The listing builds one solid part. Answer for the finished solid, in the listing's coordinates (mm). Face numbers are marked on the shaded views. A direction names the side the tool comes from. Round coordinates to 2 decimals unless told otherwise and drop trailing zeros. Loops run counter-clockwise (first coordinate to the right, second up) from the corner with the lowest first, then second, coordinate; pieces in that order, holes last. Notation, with made-up numbers: (38, 62.25) -> (45, 62.25) arc R31 ccw to (45, 99.25) -> close; hole circle Ø9 at (52.5, 72). An arc over 180 degrees is marked (long way). Use a Markdown table: item, result. Add a question column.
Q1. Section A-A on y = 25 is taken. Give the vertices of the cut face in (x, z).
Q2. For a pull along Y with two mould halves and no side action, classify the marked faces 1, 2 and 3 as released by +Y, released by -Y, zero draft, split by the parting line, or undercut.
Q3. Which of the six approach directions +Z, -Z, +X, -X, +Y, -Y give full straight-line access (tool end or side, diameter ignored) to the marked faces 4 and 5?
Q4. Consider line 1 (Y direction, x = 25, z = 22); line 2 (X direction, y = 27.5, z = 4); line 3 (X direction, y = 20, z = 5.5). Determine where each line is inside the solid, lowest interval first.
Q5. Given pin 1 Ø13.5 at (x, y) = (138.5, 74) entering from -Z; pin 2 Ø2 at (x, y) = (180, 52.5) entering from -Z; pin 3 Ø4 at (x, z) = (122.5, 8) entering from +Y; pin 4 Ø13 at (x, y) = (25, 25) entering from -Z, each flat-ended and moving along its own axis, determine where each tip first touches the part or whether it passes through.
Q6. Section C-C on x = 105 is taken. Give the vertices of the cut face in (y, z), then the cut area to 3 significant figures.
Q7. Section D-D on x = 25 is taken. Give the vertices of the cut face in (y, z).
Q8. Section B-B on z = 24.5 is taken. Give the vertices of the cut face in (x, y), then the cut area to 3 significant figures.
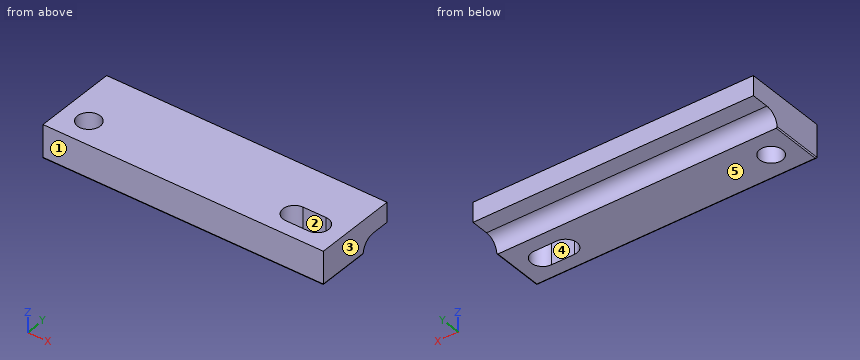
from build123d import *

# Parameters (mm, degrees)
SKETCH_1_W          = 270
SKETCH_1_H          = 80
EXTRUDE_1_DEPTH     = 32
SKETCH_2_R          = 11
CUT_EXTRUDE_1_DEPTH = 284.414890223
CUT_EXTRUDE_2_DEPTH = 284.414890223
FILLET_1_R          = 1
FILLET_2_R          = 1
FILLET_4_R          = 1


with BuildPart() as part:
    # 草图1 → 拉伸1 (new body)
    with BuildSketch(Plane.XY):
        with Locations((135, 40)):
            Rectangle(SKETCH_1_W, SKETCH_1_H)
    extrude(amount=EXTRUDE_1_DEPTH)

    # 草图2 → 切除-拉伸1 (cut, through all)
    with BuildSketch(Plane.XY.offset(32)):
        with Locations((25, 25)):
            Circle(SKETCH_2_R)
        with BuildLine():
            Line((223, 36), (245, 36))
            ThreePointArc((245, 36), (256, 25), (245, 14))
            Line((245, 14), (223, 14))
            ThreePointArc((223, 14), (212, 25), (223, 36))
        make_face()
    extrude(amount=-CUT_EXTRUDE_1_DEPTH, mode=Mode.SUBTRACT)

    # 草图3 → 切除-拉伸2 (cut, through all)
    with BuildSketch(Plane.ZY):
        with BuildLine():
            Line((13, 80), (13, 63))
            ThreePointArc((13, 63), (9.192388155, 53.807611845), (0, 50))
            Line((0, 50), (0, 80))
            Line((0, 80), (13, 80))
        make_face()
    extrude(amount=-CUT_EXTRUDE_2_DEPTH, mode=Mode.SUBTRACT)

    # 圆角1
    fillet_1_edges = [part.edges().sort_by_distance(p)[0] for p in [
        (270, 25, 0),
    ]]
    fillet(fillet_1_edges, radius=FILLET_1_R)

    # 圆角2
    fillet_2_edges = [part.edges().sort_by_distance(p)[0] for p in [
        (0, 25, 0),
    ]]
    fillet(fillet_2_edges, radius=FILLET_2_R)

    # 圆角4
    # the kernel refuses this fillet: 1 mm, written as the material it takes off along each edge
    with BuildSketch(Plane(origin=(-1.5, 0, 0), x_dir=(0, 0, 1), z_dir=(1, 0, 0))) as fillet_4_piece_1:
        with BuildLine():
            CenterArc((FILLET_4_R, -FILLET_4_R), FILLET_4_R, 90, 90)
            Line((0, -FILLET_4_R), (0, 0))
            Line((0, 0), (FILLET_4_R, 0))
        make_face()
    extrude(amount=273, mode=Mode.SUBTRACT)


solid = part.part
Checked values:
| question | item | result |
|---|---|---|
| 1 | outline | (0, 1) arc R1 ccw to (1, 0) -> (14, 0) -> (14, 32) -> (0, 32) -> close; (36, 0) -> (212, 0) -> (212, 32) -> (36, 32) -> close; (256, 0) -> (269, 0) arc R1 ccw to (270, 1) -> (270, 32) -> (256, 32) -> close |
| 2 | face 1 | released by -Y |
| 2 | face 2 | undercut |
| 2 | face 3 | zero draft |
| 3 | face 4 | +Z, -Z |
| 3 | face 5 | -Z, +X, -X, +Y, -Y |
| 4 | line 1 | y = 0 to 14, 36 to 80 |
| 4 | line 2 | x = 0 to 14.29, 35.71 to 212.29, 255.71 to 270 |
| 4 | line 3 | x = 0 to 15.2, 34.8 to 213.2, 254.8 to 270 |
| 5 | pin 1 | stops at z = 13 |
| 5 | pin 2 | stops at z = 6.06 |
| 5 | pin 3 | stops at y = 54.69 |
| 5 | pin 4 | passes through |
| 6 | outline | (0, 1) arc R1 ccw to (1, 0) -> (50, 0) arc R13 cw to (63, 13) -> (80, 13) -> (80, 32) -> (0, 32) -> close |
| 6 | area | 2,210 mm2 |
| 7 | outline | (0, 1) arc R1 ccw to (1, 0) -> (14, 0) -> (14, 32) -> (0, 32) -> close; (36, 0) -> (50, 0) arc R13 cw to (63, 13) -> (80, 13) -> (80, 32) -> (36, 32) -> close |
| 8 | outline | (0, 0) -> (270, 0) -> (270, 80) -> (0, 80) -> close; hole circle Ø22 at (25, 25); hole (223, 14) -> (245, 14) arc R11 ccw to (245, 36) -> (223, 36) arc R11 ccw to start |
| 8 | area | 20,400 mm2 |
